Autodesk Inventor part; units mm, degrees
ref_plane "YZ Plane" through (0, 0, 0) normal (1, 0, 0) x (0, 1, 0)
ref_plane "XZ Plane" through (0, 0, 0) normal (0, 1, 0) x (-1, 0, 0)
ref_plane "XY Plane" through (0, 0, 0) normal (0, 0, 1) x (1, 0, 0)
sketch "草圖1" plane through (0, 0, 0) normal (0, 0, 1) x (1, 0, 0)
  line L0 (0, 0) -> (-118.1769, -20.8378)
  line L1 (0, 0) -> (41.0424, 112.7631)
  line L2 (-150.6339, 0) -> (72.9885, 0)
  line L3 (-1.9284, 2.2981) -> (38.2199, 113.7796)
  line L4 (-1.9284, 2.2981) -> (-118.6879, -17.8816)
  line L5 (0, 0) -> (-1.9284, 2.2981) construction
  line L6 (-118.6879, -17.8816) -> (-118.1769, -20.8378)
  line L7 (38.2199, 113.7796) -> (41.0424, 112.7631)
  dimension "d0" = 10
  dimension "d1" = 70
  dimension "d2" = 120
  dimension "d3" = 60
  dimension "d5" = 3
extrude "擠出1" add sketch "草圖1" along normal blind 200
sketch "草圖2" plane through (0, 0, 200) normal (0, 0, 1) x (1, 0, 0)
  line L0 (-118.1769, -20.8378) -> (0, 0)
  line L1 (0, 0) -> (41.0424, 112.7631)
  line L2 (41.0424, 112.7631) -> (38.2199, 113.7796)
  line L3 (38.2199, 113.7796) -> (-1.9284, 2.2981)
  line L4 (-1.9284, 2.2981) -> (-118.6879, -17.8816)
  line L5 (-118.6879, -17.8816) -> (-118.1769, -20.8378)
  line L6 (-118.1769, -20.8378) -> (0, 0)
  line L7 (0, 0) -> (41.0424, 112.7631)
  line L8 (-126.8593, 28.4026) -> (-37.1114, 44.2276)
  line L9 (-37.1114, 44.2276) -> (-5.9422, 129.8641)
  line L10 (-37.1114, 44.2276) -> (0, 0) construction
  line L11 (-126.8593, 28.4026) -> (-118.1769, -20.8378)
  line L12 (-5.9422, 129.8641) -> (41.0424, 112.7631)
  dimension "d9" = 60
  dimension "d10" = 50
extrude "擠出2" add sketch "草圖2" against normal blind 200 contours L11 L8 L9 L12 L2 L3 L4 L5
shell "薄殼1" thickness 3 removed faces 4 at (-16.3319, 101.3186, 133.3333) at (25.3809, 118.4635, 133.3333) at (-67.0274, 38.9526, 133.3333) at (-123.9652, 11.9891, 133.3333)
fillet "圓角2" radius 30 4 edges at (-2.2267, 2.6537, 100) (0, 0, 100) (-37.1114, 44.2276, 198.5) (-37.1114, 44.2276, 1.5)
sketch "草圖3" plane through (0, 0, 200) normal (0, 0, 1) x (1, 0, 0)
  arc A0 (-17.0574, -3.0077) -> (5.924, 16.276) centre (-22.2668, 26.5366) ccw
  line L0 (5.924, 16.276) -> (41.0424, 112.7631)
  line L1 (41.0424, 112.7631) -> (-5.9422, 129.8641)
  line L2 (-5.9422, 129.8641) -> (-31.1874, 60.5036)
  arc A1 (-54.1687, 41.2199) -> (-31.1874, 60.5036) centre (-59.3782, 70.7642) ccw
  line L3 (-54.1687, 41.2199) -> (-126.8593, 28.4026)
  line L4 (-126.8593, 28.4026) -> (-118.1769, -20.8378)
  line L5 (-118.1769, -20.8378) -> (-17.0574, -3.0077)
  point P0 (0, 0)
properties part number "splitter"
Source: CAD feature listing. Evaluate the final solid. Frame: model axes, mm. A direction names the side the tool comes from. Give positions to 0.01 mm unless a question says otherwise; leave off trailing zeros. Loops run counter-clockwise (first coordinate to the right, second up) from the corner with the lowest first, then second, coordinate; pieces in that order, holes last. Notation, with made-up numbers: (47.5, 78) - (102.5, 78) arc R23 cw to (102.5, 99) - close; hole circle Ø4 at (-35.75, -6). An arc over 180 degrees is marked (long way). Use CSV: the item, a comma, the result in double quotes. Start each with the question number.
1. Reachability of faces 4 (the flat face through (-91.023, 34.722, 1.521)), 5 (the cylindrical face through (-5.04, 6.35, 98.64)) from +Z, -Z, +X, -X, +Y, -Y: full face, straight path, thin tool, end or side. Return the list, or none.
2. Section A-A (z = 14). Output: boundary loops of the cut face in (x, y), then the cut area to 3 significant figures.
3. Draft query along Z for faces 1 (the flat face through (-44, 39, 200)), 2 (the flat face through (-45, 41, 3)), 3 (the flat face through (-44, 39, 0)). Return one class per face: +Z half, -Z half, draft (parallel to the pull), parting line (faces both ways), or undercut.
4. Pin query (flat end, axial travel): pin 1 (3 mm diameter, centred on y = 107, z = 29, fed in from +X); pin 2 (1 mm diameter, centred on y = 89.5, z = 53.5, fed in from -X); pin 3 (10 mm diameter, centred on y = 26.5, z = 121, fed in from +X). Return the tip coordinate at first contact, or that it passes through.
5. Ray query, L1, parallel to Z at x = -54, y = 24.5; L2, parallel to Y at x = -46.5, z = 20.5; L3, parallel to Y at x = -48.5, z = 166. Return the intervals inside material, ascending.
6. Section B-B (x = -94). Output: boundary loops of the cut face in (y, z), then the cut area to 3 significant figures.
Response:
1,face 4,"+Z, -Z, -X, +Y"
1,face 5,"-X, +Y"
2,outline,"(-118.7, -17.88) - (-118.18, -20.84) - (-17.06, -3.01) arc R30 ccw to (5.92, 16.28) - (41.04, 112.76) - (38.22, 113.79) - (3.7, 18.93) arc R30 cw to (-19.28, -0.35) - close"
2,area,"715 mm²"
3,face 1,"+Z half"
3,face 2,"undercut"
3,face 3,"-Z half"
4,pin 1,"x = 39.49"
4,pin 2,"x = 29.2"
4,pin 3,"x = 11.47"
5,L1,"0 to 3, 197 to 200"
5,L2,"-8.2 to -5.15"
5,L3,"-8.55 to -5.51"
6,outline,"(-16.57, 0) - (34.2, 0) - (34.2, 3) - (-13.53, 3) - (-13.53, 197) - (34.2, 197) - (34.2, 200) - (-16.57, 200) - close"
6,area,"896 mm²"
